Source: CAD feature listing. Evaluate the final solid. Frame: model axes, mm. Face numbers are marked on the shaded views. A direction names the side the tool comes from. Round coordinates to 2 decimals unless told otherwise and drop trailing zeros. Order: outer loops, then holes, each group sorted by start corner. A loop starts at its lowest first (then second) coordinate and runs counter-clockwise, first axis right, second up. Notation, with made-up numbers: M 39.25,-38.75 L 96.25,-38.75 A15 cw 96.25,-21.75 Z; hole C 18.25,4 d7. An arc over 180 degrees is marked long. Answer as CSV lines item,"result". Start each with the question number.
Item 1: First-contact query: P1, Ø5, axis at x = -5.5, y = -5.5, coming from the +Z side; P2, Ø0.6, axis at x = 0, z = -1, coming from the +Y side; P3, Ø5, axis at y = -1, z = 23.5, coming from the -X side. Flat tips, straight axial feed; report the tip coordinate or a pass-through.
Item 2: Set-up query: the marked faces 1 and 2. Return all of +Z, -Z, +X, -X, +Y, -Y with unobstructed straight access to the full face (end or side cutting, diameter ignored); none if empty.
Item 3: Line query: line 1 (Z direction, x = 6.5, y = -4.5); line 2 (Z direction, x = 6.25, y = 7); line 3 (Z direction, x = -8.5, y = 9.75). Output: solid intervals per line, ascending. Write a range as [from, to].
Item 4: Section query A-A on z = 4.5. Return the cut outline in (x, y), plus the area to 3 significant figures.
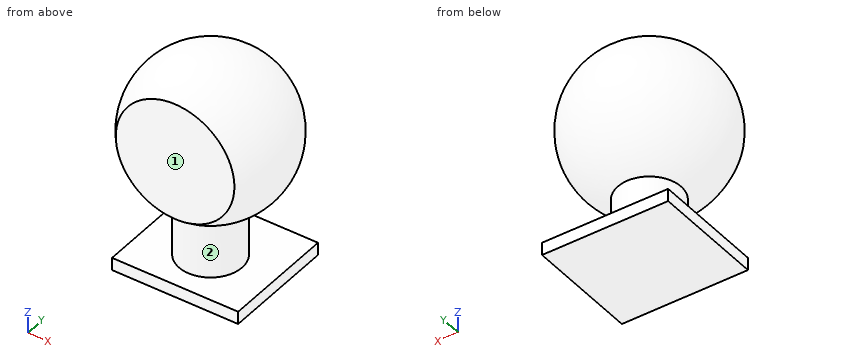
from build123d import *

# Parameters (mm, degrees)
F0_W     = 20
F0_H     = 20
F0_R     = 5
F1_DEPTH = 2
F2_DEPTH = 10
F5_W     = 20
F5_H     = 48
F6_DEPTH = 2
F5_H_2   = 50
F7_DEPTH = 5
F8_DEPTH = 2


with BuildPart() as f1:
    # F0 (on Top) → F1 (new body)
    with BuildSketch(Plane.XY):
        Rectangle(F0_W, F0_H)
        Circle(F0_R, mode=Mode.SUBTRACT)
        Circle(F0_R)
    extrude(amount=-F1_DEPTH)

    # F0 (on Top) → F2 (join)
    with BuildSketch(Plane.XY):
        Circle(F0_R)
    extrude(amount=F2_DEPTH)

    # F3 (on Right) → F4 (revolve)
    with BuildSketch(Plane.YZ):
        with BuildLine():
            Line((0, 32.42085), (0, 7.821007))
            ThreePointArc((0, 7.821007), (12.343947, 20.120929), (0, 32.42085))
        make_face()
    revolve(axis=Axis((0, 0, 16.210425), (0, 0, 1)))

    # F5 (on face) → F6 (cut)
    with BuildSketch(Plane.XZ.offset(10)):
        with Locations((0, 24)):
            Rectangle(F5_W, F5_H)
    extrude(amount=-F6_DEPTH, mode=Mode.SUBTRACT)

    # F5 (on face) → F7 (cut)
    with BuildSketch(Plane.XZ.offset(10)):
        with Locations((0, 23)):
            Rectangle(F5_W, F5_H_2)
    extrude(amount=F7_DEPTH, mode=Mode.SUBTRACT)

    # F5 (on face) → F8 (cut)
    with BuildSketch(Plane.XZ.offset(10)):
        with Locations((0, 23)):
            Rectangle(F5_W, F5_H_2)
    extrude(amount=-F8_DEPTH, mode=Mode.SUBTRACT)


solid = f1.part
Results:
1,P1,"z = 31.25"
1,P2,"y = 10"
1,P3,"x = -12.3"
2,face 1,"+Z, -Z, +X, -X, -Y"
2,face 2,"none"
3,line 1,"[-2, 0], [10.66, 29.58]"
3,line 2,"[-2, 0], [12.12, 28.12]"
3,line 3,"[-2, 0]"
4,outline,"C 0,0 d10"
4,area,"78.5 mm^2"
